Part model, mm, in its own coordinate system. Face numbers are marked on the shaded views. Round coordinates to 2 decimals unless told otherwise and drop trailing zeros. Order: outer loops, then holes, each group sorted by start corner. A loop starts at its lowest first (then second) coordinate and runs counter-clockwise, first axis right, second up. Notation, with made-up numbers: (-15.5, 88.25) -> (43.5, 88.25) arc R15 cw to (43.5, 96.25) -> close; hole circle Ø8 at (-16.75, 1). An arc over 180 degrees is marked (long way). Use CSV: the item, a comma, the result in double quotes.
Autodesk Inventor part; units mm, degrees
ref_plane "YZ Plane" through (0, 0, 0) normal (1, 0, 0) x (0, 1, 0)
ref_plane "XZ Plane" through (0, 0, 0) normal (0, 1, 0) x (-1, 0, 0)
ref_plane "XY Plane" through (0, 0, 0) normal (0, 0, 1) x (1, 0, 0)
sketch "Sketch1" plane through (0, 0, 0) normal (0, 0, 1) x (1, 0, 0)
  line L0 (-109, -87.5) -> (109, -87.5)
  line L1 (109, -87.5) -> (109, 87.5)
  line L2 (109, 87.5) -> (-109, 87.5)
  line L3 (-109, 87.5) -> (-109, -87.5)
  line L4 (-109, -87.5) -> (109, 87.5) construction
  line L5 (109, -87.5) -> (-109, 87.5) construction
  point P0 (0, 0)
  dimension "d0" = 218
  dimension "d1" = 175
extrude "Extrusion1" add sketch "Sketch1" along normal blind 28
sketch "Sketch2" plane through (0, 0, 28) normal (0, 0, 1) x (1, 0, 0)
  line L0 (-106, 84.5) -> (-66, 84.5)
  line L1 (-66, 84.5) -> (-66, 44.5)
  line L2 (-66, 44.5) -> (-106, 44.5)
  line L3 (-106, 44.5) -> (-106, 84.5)
  line L4 (-106, 84.5) -> (-66, 44.5) construction
  line L5 (-66, 84.5) -> (-106, 44.5) construction
  line L6 (109, 87.5) -> (-109, 87.5)
  line L7 (-109, 87.5) -> (-109, -87.5)
  line L8 (-63, 84.5) -> (-23, 84.5)
  line L9 (-23, 84.5) -> (-23, 44.5)
  line L10 (-23, 44.5) -> (-63, 44.5)
  line L11 (-63, 44.5) -> (-63, 84.5)
  line L12 (-63, 84.5) -> (-23, 44.5) construction
  line L13 (-23, 84.5) -> (-63, 44.5) construction
  line L14 (-20, 84.5) -> (20, 84.5)
  line L15 (20, 84.5) -> (20, 44.5)
  line L16 (20, 44.5) -> (-20, 44.5)
  line L17 (-20, 44.5) -> (-20, 84.5)
  line L18 (-20, 84.5) -> (20, 44.5) construction
  line L19 (20, 84.5) -> (-20, 44.5) construction
  line L20 (23, 84.5) -> (63, 84.5)
  line L21 (63, 84.5) -> (63, 44.5)
  line L22 (63, 44.5) -> (23, 44.5)
  line L23 (23, 44.5) -> (23, 84.5)
  line L24 (23, 84.5) -> (63, 44.5) construction
  line L25 (63, 84.5) -> (23, 44.5) construction
  line L26 (66, 84.5) -> (106, 84.5)
  line L27 (106, 84.5) -> (106, 44.5)
  line L28 (106, 44.5) -> (66, 44.5)
  line L29 (66, 44.5) -> (66, 84.5)
  line L30 (66, 84.5) -> (106, 44.5) construction
  line L31 (106, 84.5) -> (66, 44.5) construction
  line L32 (-106, 41.5) -> (-66, 41.5)
  line L33 (-66, 41.5) -> (-66, 1.5)
  line L34 (-66, 1.5) -> (-106, 1.5)
  line L35 (-106, 1.5) -> (-106, 41.5)
  line L36 (-106, 41.5) -> (-66, 1.5) construction
  line L37 (-66, 41.5) -> (-106, 1.5) construction
  line L38 (-63, 41.5) -> (-23, 41.5)
  line L39 (-23, 41.5) -> (-23, 1.5)
  line L40 (-23, 1.5) -> (-63, 1.5)
  line L41 (-63, 1.5) -> (-63, 41.5)
  line L42 (-63, 41.5) -> (-23, 1.5) construction
  line L43 (-23, 41.5) -> (-63, 1.5) construction
  line L44 (-20, 41.5) -> (20, 41.5)
  line L45 (20, 41.5) -> (20, 1.5)
  line L46 (20, 1.5) -> (-20, 1.5)
  line L47 (-20, 1.5) -> (-20, 41.5)
  line L48 (-20, 41.5) -> (20, 1.5) construction
  line L49 (20, 41.5) -> (-20, 1.5) construction
  line L50 (23, 41.5) -> (63, 41.5)
  line L51 (63, 41.5) -> (63, 1.5)
  line L52 (63, 1.5) -> (23, 1.5)
  line L53 (23, 1.5) -> (23, 41.5)
  line L54 (23, 41.5) -> (63, 1.5) construction
  line L55 (63, 41.5) -> (23, 1.5) construction
  line L56 (66, 41.5) -> (106, 41.5)
  line L57 (106, 41.5) -> (106, 1.5)
  line L58 (106, 1.5) -> (66, 1.5)
  line L59 (66, 1.5) -> (66, 41.5)
  line L60 (66, 41.5) -> (106, 1.5) construction
  line L61 (106, 41.5) -> (66, 1.5) construction
  line L62 (-106, -1.5) -> (-66, -1.5)
  line L63 (-66, -1.5) -> (-66, -41.5)
  line L64 (-66, -41.5) -> (-106, -41.5)
  line L65 (-106, -41.5) -> (-106, -1.5)
  line L66 (-106, -1.5) -> (-66, -41.5) construction
  line L67 (-66, -1.5) -> (-106, -41.5) construction
  line L68 (-63, -1.5) -> (-23, -1.5)
  line L69 (-23, -1.5) -> (-23, -41.5)
  line L70 (-23, -41.5) -> (-63, -41.5)
  line L71 (-63, -41.5) -> (-63, -1.5)
  line L72 (-63, -1.5) -> (-23, -41.5) construction
  line L73 (-23, -1.5) -> (-63, -41.5) construction
  line L74 (-20, -1.5) -> (20, -1.5)
  line L75 (20, -1.5) -> (20, -41.5)
  line L76 (20, -41.5) -> (-20, -41.5)
  line L77 (-20, -41.5) -> (-20, -1.5)
  line L78 (-20, -1.5) -> (20, -41.5) construction
  line L79 (20, -1.5) -> (-20, -41.5) construction
  line L80 (23, -1.5) -> (63, -1.5)
  line L81 (63, -1.5) -> (63, -41.5)
  line L82 (63, -41.5) -> (23, -41.5)
  line L83 (23, -41.5) -> (23, -1.5)
  line L84 (23, -1.5) -> (63, -41.5) construction
  line L85 (63, -1.5) -> (23, -41.5) construction
  line L86 (66, -1.5) -> (106, -1.5)
  line L87 (106, -1.5) -> (106, -41.5)
  line L88 (106, -41.5) -> (66, -41.5)
  line L89 (66, -41.5) -> (66, -1.5)
  line L90 (66, -1.5) -> (106, -41.5) construction
  line L91 (106, -1.5) -> (66, -41.5) construction
  line L92 (-106, -44.5) -> (-66, -44.5)
  line L93 (-66, -44.5) -> (-66, -84.5)
  line L94 (-66, -84.5) -> (-106, -84.5)
  line L95 (-106, -84.5) -> (-106, -44.5)
  line L96 (-106, -44.5) -> (-66, -84.5) construction
  line L97 (-66, -44.5) -> (-106, -84.5) construction
  line L98 (-63, -44.5) -> (-23, -44.5)
  line L99 (-23, -44.5) -> (-23, -84.5)
  line L100 (-23, -84.5) -> (-63, -84.5)
  line L101 (-63, -84.5) -> (-63, -44.5)
  line L102 (-63, -44.5) -> (-23, -84.5) construction
  line L103 (-23, -44.5) -> (-63, -84.5) construction
  line L104 (-20, -44.5) -> (20, -44.5)
  line L105 (20, -44.5) -> (20, -84.5)
  line L106 (20, -84.5) -> (-20, -84.5)
  line L107 (-20, -84.5) -> (-20, -44.5)
  line L108 (-20, -44.5) -> (20, -84.5) construction
  line L109 (20, -44.5) -> (-20, -84.5) construction
  line L110 (23, -44.5) -> (63, -44.5)
  line L111 (63, -44.5) -> (63, -84.5)
  line L112 (63, -84.5) -> (23, -84.5)
  line L113 (23, -84.5) -> (23, -44.5)
  line L114 (23, -44.5) -> (63, -84.5) construction
  line L115 (63, -44.5) -> (23, -84.5) construction
  line L116 (66, -44.5) -> (106, -44.5)
  line L117 (106, -44.5) -> (106, -84.5)
  line L118 (106, -84.5) -> (66, -84.5)
  line L119 (66, -84.5) -> (66, -44.5)
  line L120 (66, -44.5) -> (106, -84.5) construction
  line L121 (106, -44.5) -> (66, -84.5) construction
  point P0 (0, 0)
  point P1 (-86, 64.5)
  point P2 (-43, 64.5)
  point P3 (0, 64.5)
  point P4 (43, 64.5)
  point P5 (86, 64.5)
  point P6 (-86, 21.5)
  point P7 (-43, 21.5)
  point P8 (0, 21.5)
  point P9 (43, 21.5)
  point P10 (86, 21.5)
  point P11 (-86, -21.5)
  point P12 (-43, -21.5)
  point P13 (0, -21.5)
  point P14 (43, -21.5)
  point P15 (86, -21.5)
  point P16 (-86, -64.5)
  point P17 (-43, -64.5)
  point P18 (0, -64.5)
  point P19 (43, -64.5)
  point P20 (86, -64.5)
  dimension "d4" = 40
  dimension "d5" = 3
  dimension "d6" = 3
  dimension "d7" = 40
  dimension "d10" = 43
  dimension "d13" = 43
extrude "Extrusion2" cut sketch "Sketch2" against normal blind 25
equation "\"d0\" = box_length"
equation "\"d1\" = box_width"
equation "\"d2\" = hole_height + wall"
equation "\"d4\" = hole"
equation "\"d5\" = wall"
equation "\"d6\" = wall"
equation "\"d7\" = hole"
equation "\"d10\" = hole + wall"
equation "\"d13\" = hole + wall"
equation "\"d16\" = hole_height"
equation "\"hole\" = 40"
equation "\"wall\" = 3"
equation "\"hole_height\" = 25"
properties part number "RatPelletBox_v01"
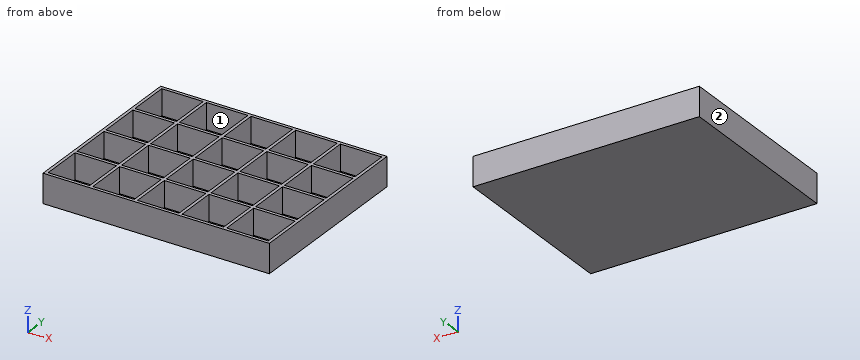
(1) Drop a flat-ended pin along its axis: P1, Ø12, axis at x = 80, y = 67, coming from the +Z side. Give the stop position or say it passes through.
Reply:
P1,"z = 3"
(2) Cut at B-B, the plane x = 10. Give the cut face in (y, z), then the cut area to 3 significant figures.
Reply:
outline,"(-87.5, 0) -> (87.5, 0) -> (87.5, 28) -> (84.5, 28) -> (84.5, 3) -> (44.5, 3) -> (44.5, 28) -> (41.5, 28) -> (41.5, 3) -> (1.5, 3) -> (1.5, 28) -> (-1.5, 28) -> (-1.5, 3) -> (-41.5, 3) -> (-41.5, 28) -> (-44.5, 28) -> (-44.5, 3) -> (-84.5, 3) -> (-84.5, 28) -> (-87.5, 28) -> close"
area,"900 mm2"
(3) Cut at C-C, the plane z = 16. State how many separate pieces and enclosed holes the cut face has, then the cut area to 3 significant figures.
Reply:
separate pieces,"1"
enclosed holes,"20"
area,"6,150 mm2"
(4) Probe probe 1 along Y at (x, z) = (34, 9.5); probe 2 along X at (y, z) = (-55, 14.25); probe 3 along Z at (x, y) = (-71, -71). List the from-to ranges inside material, lowest first. Write a range as [from, to].
Reply:
probe 1,"[-87.5, -84.5], [-44.5, -41.5], [-1.5, 1.5], [41.5, 44.5], [84.5, 87.5]"
probe 2,"[-109, -106], [-66, -63], [-23, -20], [20, 23], [63, 66], [106, 109]"
probe 3,"[0, 3]"
(5) Cut at A-A, the plane y = 48. Give the cut face in (x, z), then the cut area to 3 significant figures.
Reply:
outline,"(-109, 0) -> (109, 0) -> (109, 28) -> (106, 28) -> (106, 3) -> (66, 3) -> (66, 28) -> (63, 28) -> (63, 3) -> (23, 3) -> (23, 28) -> (20, 28) -> (20, 3) -> (-20, 3) -> (-20, 28) -> (-23, 28) -> (-23, 3) -> (-63, 3) -> (-63, 28) -> (-66, 28) -> (-66, 3) -> (-106, 3) -> (-106, 28) -> (-109, 28) -> close"
area,"1,100 mm2"
(6) Pull direction X, two halves, no side cores. Call the marked faces 1 and 2: released by +X, released by -X, zero draft, split by the parting line, or undercut.
Reply:
face 1,"undercut"
face 2,"released by -X"
